Part model, mm, in its own coordinate system. Give positions to 0.01 mm unless a question says otherwise; leave off trailing zeros. Order: outer loops, then holes, each group sorted by start corner. A loop starts at its lowest first (then second) coordinate and runs counter-clockwise, first axis right, second up. Notation, with made-up numbers: (38.5, -14.5) -> (56.5, -14.5) arc R18 ccw to (56.5, -1.5) -> close; hole circle Ø10 at (-3.5, 87). An arc over 180 degrees is marked (long way). Write item = value, one per line. Start each with the question number.
Item 1: Band-saw the part on A-A on z = 0. Write the cut outline in (x, y).
Item 2: Band-saw the part on B-B on x = 0. Write the cut outline in (y, z), plus the area to 3 significant figures.
Item 3: Drill centre lines: line 1 along X through (y, z) = (-0.05, -94); line 2 along Z through (x, y) = (123, -0.05); line 3 along X through (y, z) = (-0.05, 0). Where is each one in solid material? Low to high.
Item 4: Flat gauge pin, fed straight in: P1, Ø7, axis at x = 0, z = 0, coming from the -Y side. Where does the tip first touch, or does it go through?
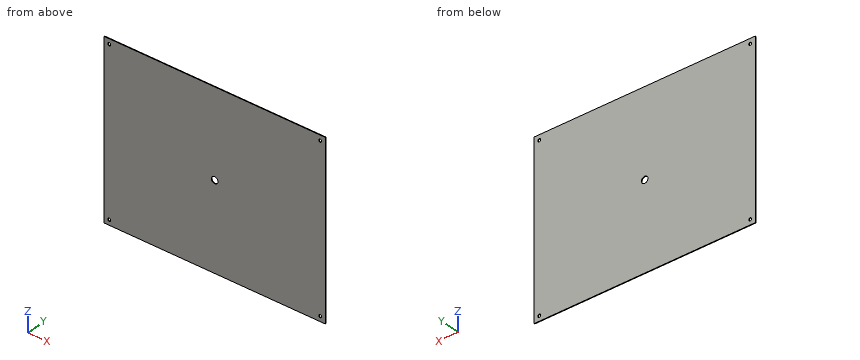
```python
from build123d import *

# Parameters (mm, degrees)
BOSS_EXTRUDE1_DEPTH      = 152.4
BOSS_EXTRUDE1_DEPTH_BACK = 152.4
SKETCH3_W                = 304.8
SKETCH3_H                = 0.79375
SKETCH4_OUTSIDE_W        = 393.01
SKETCH4_OUTSIDE_H        = 393.01
SKETCH4_OUTSIDE_W_2      = 258
SKETCH4_OUTSIDE_H_2      = 200
FIT2ENCLOSURE_DEPTH      = 0.79375
CUBEMOUNTHOLES_D         = 3.4
DRAINHOLE_REACH          = 165.223
SKETCH8_R                = 3.81


with BuildPart() as part:
    # Sketch3 → Boss-Extrude1 (new, two sides: drawn at the far end of the back side and taken through both)
    with BuildSketch(Plane.XY.offset(-BOSS_EXTRUDE1_DEPTH_BACK)):
        Rectangle(SKETCH3_W, SKETCH3_H)
    extrude(amount=BOSS_EXTRUDE1_DEPTH + BOSS_EXTRUDE1_DEPTH_BACK)

    # Sketch4 outside → Fit2Enclosure (cut)
    with BuildSketch(Plane(origin=(0, 0.396875, 0), x_dir=(1, 0, 0), z_dir=(0, 1, 0))):
        Rectangle(SKETCH4_OUTSIDE_W, SKETCH4_OUTSIDE_H)
        Rectangle(SKETCH4_OUTSIDE_W_2, SKETCH4_OUTSIDE_H_2, mode=Mode.SUBTRACT)
    extrude(amount=-FIT2ENCLOSURE_DEPTH, mode=Mode.SUBTRACT)

    # CubeMountHoles (through all)
    with Locations(Plane(origin=(0, 0.396875, 0), x_dir=(1, 0, 0), z_dir=(0, 1, 0))):
        with Locations((-123, 94), (123, 94), (123, -94), (-122.975, -94)):
            Hole(CUBEMOUNTHOLES_D / 2)

    # Sketch8 → DrainHole (cut, up to next)
    with BuildSketch(Plane(origin=(0, 0.396875, 0), x_dir=(1, 0, 0), z_dir=(0, 1, 0)), mode=Mode.PRIVATE) as drainhole_sk1:
        with Locations(Location((0, 0, 0), (0, 0, 270))):
            Circle(SKETCH8_R)
    drainhole_tool1 = extrude(drainhole_sk1.sketch, amount=-DRAINHOLE_REACH, mode=Mode.PRIVATE) & part.part
    add(drainhole_tool1.solids().sort_by_distance((0, 0.396875, 0))[0], mode=Mode.SUBTRACT)


solid = part.part
```
Values found:
q1.outline = (-129, -0.4) -> (-3.81, -0.4) -> (-3.81, 0.4) -> (-129, 0.4) -> close; (3.81, -0.4) -> (129, -0.4) -> (129, 0.4) -> (3.81, 0.4) -> close
q2.outline = (-0.4, -100) -> (0.4, -100) -> (0.4, -3.81) -> (-0.4, -3.81) -> close; (-0.4, 3.81) -> (0.4, 3.81) -> (0.4, 100) -> (-0.4, 100) -> close
q2.area = 153 mm^2
q3.line_1 = -129 to -124.7, -121.3 to 121.3, 124.7 to 129
q3.line_2 = -100 to -95.7, -92.3 to 92.3, 95.7 to 100
q3.line_3 = -129 to -3.81, 3.81 to 129
q4.P1 = through
